from build123d import *

# Parameters (mm, degrees)
BOSS_EXTRUDE1_DEPTH = 1.5
BOSS_EXTRUDE2_DEPTH = 2
SKETCH3_W           = 80.4
SKETCH3_H           = 88.4
CUT_EXTRUDE1_DEPTH  = 2
SKETCH4_R           = 9
CUT_EXTRUDE2_DEPTH  = 2
SKETCH5_R           = 1.75
SKETCH5_R_2         = 2.75
CUT_EXTRUDE3_DEPTH  = 2
SKETCH6_R           = 6.5
CUT_EXTRUDE4_DEPTH  = 2


with BuildPart() as part:
    # Sketch1 → Boss-Extrude1 (new body)
    with BuildSketch(Plane(origin=(0, 0, 0), x_dir=(1, 0, 0), z_dir=(0, 1, 0))):
        with BuildLine():
            Line((3, 0), (86, 0))
            ThreePointArc((86, 0), (88.121320344, 0.878679656), (89, 3))
            Line((89, 3), (89, 94))
            ThreePointArc((89, 94), (88.121320344, 96.121320344), (86, 97))
            Line((86, 97), (3, 97))
            ThreePointArc((3, 97), (0.878679656, 96.121320344), (0, 94))
            Line((0, 94), (0, 3))
            ThreePointArc((0, 3), (0.878679656, 0.878679656), (3, 0))
        make_face()
    extrude(amount=BOSS_EXTRUDE1_DEPTH)

    # Sketch2 → Boss-Extrude2 (add)
    with BuildSketch(Plane(origin=(0, 1.5, 0), x_dir=(1, 0, 0), z_dir=(0, 1, 0))):
        with BuildLine():
            Line((2.3, 94), (2.3, 3))
            ThreePointArc((2.3, 3), (2.505025253, 2.505025253), (3, 2.3))
            Line((3, 2.3), (86, 2.3))
            ThreePointArc((86, 2.3), (86.494974747, 2.505025253), (86.7, 3))
            Line((86.7, 3), (86.7, 94))
            ThreePointArc((86.7, 94), (86.494974747, 94.494974747), (86, 94.7))
            Line((86, 94.7), (3, 94.7))
            ThreePointArc((3, 94.7), (2.505025253, 94.494974747), (2.3, 94))
        make_face()
    extrude(amount=BOSS_EXTRUDE2_DEPTH)

    # Sketch3 → Cut-Extrude1 (cut)
    with BuildSketch(Plane(origin=(0, 3.5, 0), x_dir=(1, 0, 0), z_dir=(0, 1, 0))):
        with Locations((44.5, 48.5)):
            Rectangle(SKETCH3_W, SKETCH3_H)
    extrude(amount=-CUT_EXTRUDE1_DEPTH, mode=Mode.SUBTRACT)

    # Sketch4 → Cut-Extrude2 (cut)
    with BuildSketch(Plane(origin=(0, 1.5, 0), x_dir=(1, 0, 0), z_dir=(0, 1, 0))):
        with Locations((31.5, 48.5)):
            Circle(SKETCH4_R)
        with Locations((57.5, 48.5)):
            Circle(SKETCH4_R)
    extrude(amount=-CUT_EXTRUDE2_DEPTH, mode=Mode.SUBTRACT)

    # Sketch5 → Cut-Extrude3 (cut)
    with BuildSketch(Plane(origin=(0, 1.5, 0), x_dir=(1, 0, 0), z_dir=(0, 1, 0))):
        with Locations((29.3, 80.7)):
            Circle(SKETCH5_R)
        with Locations((50.2, 80.7)):
            Circle(SKETCH5_R_2)
    extrude(amount=-CUT_EXTRUDE3_DEPTH, mode=Mode.SUBTRACT)

    # Sketch6 → Cut-Extrude4 (cut)
    with BuildSketch(Plane(origin=(0, 1.5, 0), x_dir=(1, 0, 0), z_dir=(0, 1, 0))):
        with Locations((44.5, 22.3)):
            Circle(SKETCH6_R)
    extrude(amount=-CUT_EXTRUDE4_DEPTH, mode=Mode.SUBTRACT)


solid = part.part
Read the model definition and answer for the solid it produces. Units are mm, in the model's axes. A direction names the side the tool comes from. Round coordinates to 2 decimals unless told otherwise and drop trailing zeros. Loops run counter-clockwise (first coordinate to the right, second up) from the corner with the lowest first, then second, coordinate; pieces in that order, holes last.
Q1. Section C-C on x = 17.5 is taken. Write down the section's boundary in (y, z).
Q2. Which of the six approach directions +Z, -Z, +X, -X, +Y, -Y give full straight-line access (tool end or side, diameter ignored) to faces 1 (the face through (84.7, 3, -48)), 2 (the face through (30.328, 0.76, -57.423)), 3 (the face through (2.3, 2, -49))?
Q3. Determine the mould class of faces 4 (the face through (44, 3, -4.3)), 5 (the face through (0.86, 0.74, -0.9)), 6 (the face through (88.14, 0.74, -96.1)) for opening direction Z: released by +Z, released by -Z, zero draft, split by the parting line, or undercut.
Q4. Section A-A on x = 57.5 is taken. Write down the section's boundary in (y, z).
Q5. Section D-D on z = -64 is taken. Write down the section's boundary in (x, y).
Q6. Each of these flat-tipped pins is pushed along its axis until it touches: pin 1 (5.5 mm diameter, centred on x = 29.3, z = -80.7, fed in from -Y); pin 2 (15 mm diameter, centred on x = 44.5, z = -22.3, fed in from +Y); pin 3 (0.6 mm diameter, centred on y = 2.5, z = -38, fed in from -X); pin 4 (1.6 mm diameter, centred on y = 3, z = -68, fed in from +X). Where does it stop, or does it pass through?
Q7. Consider probe 1 along X at (y, z) = (0.45, -48.5); probe 2 along X at (y, z) = (0.7, -50); probe 3 along X at (y, z) = (3.1, -76). Determine where each line is inside the solid, lowest interval first.
Q8. Section B-B on z = -48.5 is taken. Write down the section's boundary in (x, y).
Output:
1. outline: (0, -97) - (1.5, -97) - (1.5, -94.7) - (3.5, -94.7) - (3.5, -92.7) - (1.5, -92.7) - (1.5, -4.3) - (3.5, -4.3) - (3.5, -2.3) - (1.5, -2.3) - (1.5, 0) - (0, 0) - close
2. face 1: +Y
2. face 2: +Y, -Y
2. face 3: +Z, -Z, -X, +Y
3. face 4: undercut
3. face 5: released by +Z
3. face 6: released by -Z
4. outline: (0, -97) - (1.5, -97) - (1.5, -94.7) - (3.5, -94.7) - (3.5, -92.7) - (1.5, -92.7) - (1.5, -57.5) - (0, -57.5) - close; (0, -39.5) - (1.5, -39.5) - (1.5, -4.3) - (3.5, -4.3) - (3.5, -2.3) - (1.5, -2.3) - (1.5, 0) - (0, 0) - close
5. outline: (0, 0) - (89, 0) - (89, 1.5) - (86.7, 1.5) - (86.7, 3.5) - (84.7, 3.5) - (84.7, 1.5) - (4.3, 1.5) - (4.3, 3.5) - (2.3, 3.5) - (2.3, 1.5) - (0, 1.5) - close
6. pin 1: stops at y = 0
6. pin 2: stops at y = 1.5
6. pin 3: stops at x = 2.3
6. pin 4: stops at x = 86.7
7. probe 1: x = 0 to 22.5, 40.5 to 48.5, 66.5 to 89
7. probe 2: x = 0 to 22.63, 40.37 to 48.63, 66.37 to 89
7. probe 3: x = 2.3 to 4.3, 84.7 to 86.7
8. outline: (0, 0) - (22.5, 0) - (22.5, 1.5) - (4.3, 1.5) - (4.3, 3.5) - (2.3, 3.5) - (2.3, 1.5) - (0, 1.5) - close; (40.5, 0) - (48.5, 0) - (48.5, 1.5) - (40.5, 1.5) - close; (66.5, 0) - (89, 0) - (89, 1.5) - (86.7, 1.5) - (86.7, 3.5) - (84.7, 3.5) - (84.7, 1.5) - (66.5, 1.5) - close
